Can you work these out from the model? Positions are in its coordinate system, mm. Face numbers are marked on the shaded views. A direction names the side the tool comes from. Coordinates: 2 decimals unless noted, no trailing zeros. Order: outer loops, then holes, each group sorted by start corner. A loop starts at its lowest first (then second) coordinate and runs counter-clockwise, first axis right, second up. Notation, with made-up numbers: (68.25, 62.5) -> (120.25, 62.5) arc R20 ccw to (120.25, 84.5) -> close; hole circle Ø3 at (3.25, 3.25). An arc over 180 degrees is marked (long way). Answer in a Markdown table with one row per item.
```python
from build123d import *

# Parameters (mm, degrees)
SKETCH1_R           = 28.5
SKETCH1_R_2         = 15
BOSS_EXTRUDE1_DEPTH = 38
SKETCH2_W           = 57
SKETCH2_H           = 84
BOSS_EXTRUDE2_DEPTH = 16
SKETCH6_W           = 57
SKETCH6_H           = 38
BOSS_EXTRUDE4_DEPTH = 14
SKETCH7_W           = 57
SKETCH7_H           = 38
BOSS_EXTRUDE5_DEPTH = 14
SKETCH8_R           = 8
CUT_EXTRUDE3_DEPTH  = 104.847243584
CUT_EXTRUDE4_DEPTH  = 104.847243584
CUT_EXTRUDE5_START  = -38
CUT_EXTRUDE5_DEPTH  = 38


with BuildPart() as part:
    # Sketch1 → Boss-Extrude1 (new body)
    with BuildSketch(Plane(origin=(0, 0, 0), x_dir=(1, 0, 0), z_dir=(0, 1, 0))):
        with Locations(Location((0, 0, 0), (0, 0, 270))):
            Circle(SKETCH1_R)
        with Locations(Location((0, 0, 0), (0, 0, 270))):
            Circle(SKETCH1_R_2, mode=Mode.SUBTRACT)
    extrude(amount=BOSS_EXTRUDE1_DEPTH)

    # Sketch2 → Boss-Extrude2 (add)
    with BuildSketch(Plane.XZ):
        Rectangle(SKETCH2_W, SKETCH2_H)
    extrude(amount=BOSS_EXTRUDE2_DEPTH)

    # Sketch6 → Boss-Extrude4 (add)
    with BuildSketch(Plane.XY.offset(42)):
        with Locations((0, -35)):
            Rectangle(SKETCH6_W, SKETCH6_H)
    extrude(amount=-BOSS_EXTRUDE4_DEPTH)

    # Sketch7 → Boss-Extrude5 (add)
    with BuildSketch(Plane(origin=(0, 0, -42), x_dir=(-1, 0, 0), z_dir=(0, 0, -1))):
        with Locations((0, -35)):
            Rectangle(SKETCH7_W, SKETCH7_H)
    extrude(amount=-BOSS_EXTRUDE5_DEPTH)

    # Sketch8 → Cut-Extrude3 (cut, through all)
    with BuildSketch(Plane(origin=(0, 0, -42), x_dir=(-1, 0, 0), z_dir=(0, 0, -1))):
        with Locations((0, -34)):
            Circle(SKETCH8_R)
    extrude(amount=-CUT_EXTRUDE3_DEPTH, mode=Mode.SUBTRACT)

    # Sketch9 → Cut-Extrude4 (cut, through all)
    with BuildSketch(Plane.XY.offset(42)):
        with BuildLine():
            Line((-19.473528625, -38.558693112), (-28.5, 0))
            Line((-28.5, 0), (-28.5, -54))
            Line((-28.5, -54), (0, -54))
            ThreePointArc((0, -54), (-12.42630552, -49.671213454), (-19.473528625, -38.558693112))
        make_face()
        with BuildLine():
            ThreePointArc((19.473522225, -38.558720453), (12.426294519, -49.671222177), (0, -54))
            Line((0, -54), (28.5, -54))
            Line((28.5, -54), (28.5, 0))
            Line((28.5, 0), (19.473522225, -38.558720453))
        make_face()
    extrude(amount=-CUT_EXTRUDE4_DEPTH, mode=Mode.SUBTRACT)

    # Sketch11 → Cut-Extrude5 (cut)
    with BuildSketch(Plane(origin=(0, 38, 0), x_dir=(1, 0, 0), z_dir=(0, 1, 0)).offset(CUT_EXTRUDE5_START)):
        with BuildLine():
            Line((-4, 17.956832295), (4, 17.956832295))
            Line((4, 17.956832295), (4, 14.456832295))
            ThreePointArc((4, 14.456832295), (0, 15), (-4, 14.456832295))
            Line((-4, 14.456832295), (-4, 17.956832295))
        make_face()
    extrude(amount=CUT_EXTRUDE5_DEPTH, mode=Mode.SUBTRACT)


solid = part.part
```
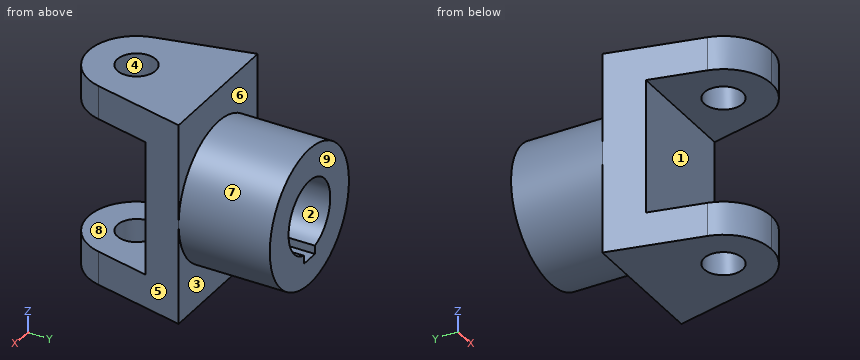
(1) We'd pull the mould along Y, two halves only. Please class the marked faces 1, 2, 3 and 4: +Y half, -Y half, draft (parallel to the pull), parting line (faces both ways), or undercut.
Response values:
| item | result |
|---|---|
| face 1 | -Y half |
| face 2 | draft |
| face 3 | +Y half |
| face 4 | undercut |
(2) I need wall thicknesses on line 1 (X direction, y = 23.5, z = 0); line 2 (Y direction, x = 0, z = -33); line 3 (Z direction, x = -13.5, y = -23). Which ranges of each line are inside material? Lowest first, please. Write a range as [from, to].
Response values:
| item | result |
|---|---|
| line 1 | [-28.5, -15], [15, 28.5] |
| line 2 | [-54, -42], [-26, 0] |
| line 3 | [-42, -28], [28, 42] |
(3) Suppose I cut it at D-D (x = 6). Please give me the cut outline in (y, z).
Response values:
| item | result |
|---|---|
| outline | (-53.08, -42) -> (-39.29, -42) -> (-39.29, -28) -> (-53.08, -28) -> close; (-53.08, 28) -> (-39.29, 28) -> (-39.29, 42) -> (-53.08, 42) -> close; (-28.71, -42) -> (0, -42) -> (0, -27.86) -> (38, -27.86) -> (38, -13.75) -> (0, -13.75) -> (0, 13.75) -> (38, 13.75) -> (38, 27.86) -> (0, 27.86) -> (0, 42) -> (-28.71, 42) -> (-28.71, 28) -> (-16, 28) -> (-16, -28) -> (-28.71, -28) -> close |
(4) Will these pins go through, and if not, where does the flat tip stop? pin 1 Ø18.5 at (x, y) = (0, -34) entering from -Z; pin 2 Ø2 at (x, z) = (19, -25.5) entering from +Y; pin 3 Ø2 at (y, z) = (-8, 8.5) entering from +X; pin 4 Ø1.1 at (y, z) = (22.5, -16.5) entering from +X.
Response values:
| item | result |
|---|---|
| pin 1 | z = -42 |
| pin 2 | y = 0 |
| pin 3 | x = 26.86 |
| pin 4 | x = 23.62 |
(5) Suppose I cut it at B-B (x = 16.5). Please give me the cut outline in (y, z).
Response values:
| item | result |
|---|---|
| outline | (-45.3, -42) -> (0, -42) -> (0, -23.24) -> (38, -23.24) -> (38, 23.24) -> (0, 23.24) -> (0, 42) -> (-45.3, 42) -> (-45.3, 28) -> (-16, 28) -> (-16, -28) -> (-45.3, -28) -> close |
(6) Suppose I cut it at C-C (z = 12). Please give me the cut outline in (x, y), and give its area (3 significant figures).
Response values:
| item | result |
|---|---|
| outline | (-28.5, 0) -> (-24.75, -16) -> (24.75, -16) -> (28.5, 0) -> (25.85, 0) -> (25.85, 38) -> (9, 38) -> (9, 0) -> (-9, 0) -> (-9, 38) -> (-25.85, 38) -> (-25.85, 0) -> close |
| area | 2,130 mm2 |
(7) Suppose I cut it at A-A (z = 36). Please give me the cut outline in (x, y).
Response values:
| item | result |
|---|---|
| outline | (-28.5, 0) -> (-19.47, -38.56) arc R20 ccw to (19.47, -38.56) -> (28.5, 0) -> close; hole circle Ø16 at (0, -34) |
(8) On a 3-axis mill with a long thin cutter (end or side, diameter ignored), from which of +Z, -Z, +X, -X, +Y, -Y can I reach the whole of each face in a straight line? I mean the marked faces 5, 6, 7, 8 and 9. Say none if no direction works.
Response values:
| item | result |
|---|---|
| face 5 | +Z, -Z, +X, -Y |
| face 6 | +Z, +Y |
| face 7 | +Y |
| face 8 | +X, -X, -Y |
| face 9 | +Z, -Z, +X, -X, +Y |
